from build123d import *

# Parameters (mm, degrees)
PAD_DEPTH        = 3
HOLE_D           = 3.5
HOLE_CSINK_D     = 7
HOLE_CSINK_ANGLE = 90
CHAMFER_SIZE     = 1
SKETCH002_W      = 31
SKETCH002_H      = 47
POCKET_DEPTH     = 2.2
SKETCH003_W      = 28
SKETCH003_H      = 47
POCKET001_DEPTH  = 3.001
POCKET002_DEPTH  = 3.001
CHAMFER001_SIZE  = 0.5
PAD001_DEPTH     = 15


with BuildPart() as part:
    # Sketch → Pad (new body)
    with BuildSketch(Plane.XY):
        with BuildLine():
            Line((6, 0), (46.1, 0))
            ThreePointArc((46.1, 0), (50.342641, 1.757359), (52.1, 6))
            Line((52.1, 6), (52.1, 62))
            ThreePointArc((52.1, 62), (50.342641, 66.242641), (46.1, 68))
            Line((46.1, 68), (6, 68))
            ThreePointArc((6, 68), (1.757359, 66.242641), (0, 62))
            Line((0, 62), (0, 6))
            ThreePointArc((0, 6), (1.757359, 1.757359), (6, 0))
        make_face()
    extrude(amount=PAD_DEPTH)

    # Hole (through all)
    with Locations(Plane(origin=(0, 0, 0), x_dir=(1, 0, 0), z_dir=(0, 0, -1))):
        with Locations((6, -52.65), (46.1, -52.65), (46.1, -15.35), (6, -15.35)):
            CounterSinkHole(HOLE_D / 2, HOLE_CSINK_D / 2, counter_sink_angle=HOLE_CSINK_ANGLE)

    # Chamfer
    chamfer_edges = [part.edges().sort_by_distance(p)[0] for p in [
        (52.1, 34, 0),
    ]]
    chamfer(chamfer_edges, length=CHAMFER_SIZE)

    # Sketch002 (on DatumPlane) → Pocket (cut)
    with BuildSketch(Plane.XY.offset(3)):
        with Locations((26.05, 27)):
            Rectangle(SKETCH002_W, SKETCH002_H)
    extrude(amount=-POCKET_DEPTH, mode=Mode.SUBTRACT)

    # Sketch003 (on DatumPlane) → Pocket001 (cut, through all)
    with BuildSketch(Plane.XY.offset(3)):
        with Locations((26.05, 27)):
            Rectangle(SKETCH003_W, SKETCH003_H)
    extrude(amount=-POCKET001_DEPTH, mode=Mode.SUBTRACT)

    # Sketch004 (on DatumPlane) → Pocket002 (cut, through all)
    with BuildSketch(Plane.XY.offset(3)):
        with BuildLine():
            Line((11.05, 54.5), (11.05, 65.5))
            ThreePointArc((11.55, 66), (11.196447, 65.853553), (11.05, 65.5))
            Line((11.55, 66), (40.55, 66))
            ThreePointArc((41.05, 65.5), (40.903553, 65.853553), (40.55, 66))
            Line((41.05, 65.5), (41.05, 54.5))
            ThreePointArc((40.55, 54), (40.903553, 54.146447), (41.05, 54.5))
            Line((40.55, 54), (11.55, 54))
            ThreePointArc((11.05, 54.5), (11.196447, 54.146447), (11.55, 54))
        make_face()
    extrude(amount=-POCKET002_DEPTH, mode=Mode.SUBTRACT)

    # Chamfer001
    chamfer001_edges = [part.edges().sort_by_distance(p)[0] for p in [
        (26.05, 54, 0),
        (26.05, 54, 3),
    ]]
    chamfer(chamfer001_edges, length=CHAMFER001_SIZE)

    # Sketch005 (on DatumPlane) → Pad001 (join)
    with BuildSketch(Plane.XY.offset(3)):
        with BuildLine():
            Line((10.05, 52.5), (10.05, 51.5))
            ThreePointArc((10.05, 51.5), (10.342893, 50.792893), (11.05, 50.5))
            Line((11.05, 50.5), (41.05, 50.5))
            ThreePointArc((41.05, 50.5), (41.757107, 50.792893), (42.05, 51.5))
            Line((42.05, 51.5), (42.05, 52.5))
            ThreePointArc((42.05, 52.5), (41.757107, 53.207107), (41.05, 53.5))
            Line((41.05, 53.5), (11.05, 53.5))
            ThreePointArc((11.05, 53.5), (10.342893, 53.207107), (10.05, 52.5))
        make_face()
    extrude(amount=PAD001_DEPTH)


solid = part.part
Verification items for the finished model (mm, model axes). A direction names the side the tool comes from. Give positions to 0.01 mm unless a question says otherwise; leave off trailing zeros. Write each loop counter-clockwise with the first axis right and the second up, starting at its lowest first coordinate (ties: lowest second). Pieces come first, ordered by that corner, then holes. Notation, with made-up numbers: M 66.5,35.5 L 109.5,35.5 A18 cw 109.5,57.5 Z; hole C 44.25,45.25 d6. An arc over 180 degrees is marked long. Use CSV: the item, a comma, the result in double quotes.
1) Cross-section at C-C (z = 9). Enter the section's corners in (x, y).
Final values:
outline,"M 10.05,51.5 A1 ccw 11.05,50.5 L 41.05,50.5 A1 ccw 42.05,51.5 L 42.05,52.5 A1 ccw 41.05,53.5 L 11.05,53.5 A1 ccw 10.05,52.5 Z"
2) Cross-section at A-A (x = 24). Enter the section's corners in (y, z), plus the area to 3 significant figures.
Final values:
outline,"M 0,1 L 1,0 L 3.5,0 L 3.5,3 L 0,3 Z; M 50.5,0 L 53.5,0 L 54,0.5 L 54,2.5 L 53.5,3 L 53.5,18 L 50.5,18 Z; M 66,0.5 L 66.5,0 L 67,0 L 68,1 L 68,3 L 66.5,3 L 66,2.5 Z"
area,"70.5 mm²"
3) Go/stop test with flat-tipped pins: pin 1 Ø1 at (x, y) = (45, 54) entering from +Z; pin 2 Ø8 at (y, z) = (47.5, 11.5) entering from +X; pin 3 Ø10 at (x, z) = (41.5, 14) entering from +Y; pin 4 Ø10 at (x, z) = (42.5, 7) entering from +Y. Record where each tip stops, or that it passes through.
Final values:
pin 1,"z = 3"
pin 2,"x = 42.05"
pin 3,"y = 53.5"
pin 4,"y = 68"
4) Release check for a two-part mould opening along X. For faces 4 (the face through (26, 68, 2)), 5 (the face through (49.868, 65.686, 0.271)), 6 (the face through (6.38, 54.36, 2.38)) record: released by +X, released by -X, zero draft, split by the parting line, or undercut.
Final values:
face 4,"zero draft"
face 5,"released by +X"
face 6,"undercut"
5) Material ranges on line 1 along X through (y, z) = (52.65, 2.15); line 2 along Y through (x, z) = (46.1, 2.2); line 3 along X through (y, z) = (15.35, 2.3), recorded low to high.
Final values:
line 1,"0 to 4.25, 7.75 to 44.35, 47.85 to 52.1"
line 2,"0 to 13.6, 17.1 to 50.9, 54.4 to 68"
line 3,"0 to 4.25, 7.75 to 10.55, 41.55 to 44.35, 47.85 to 52.1"
6) Access from +Z, -Z, +X, -X, +Y, -Y to the whole of each face (thin tool, end or side, straight path). Record for faces 1 (the face through (1.804, 66.289, 1.986)), 2 (the face through (26, 66, 2)), 3 (the face through (10.55, 27, 2)).
Final values:
face 1,"+Z, -Z, -X, +Y"
face 2,"+Z, -Z"
face 3,"+Z"
7) Cross-section at B-B (y = 15.35). Enter the section's corners in (x, z), plus the area to 3 significant figures.
Final values:
outline,"M 0,1 L 1,0 L 2.5,0 L 4.25,1.75 L 4.25,3 L 0,3 Z; M 7.75,1.75 L 9.5,0 L 12.05,0 L 12.05,0.8 L 10.55,0.8 L 10.55,3 L 7.75,3 Z; M 40.05,0 L 42.6,0 L 44.35,1.75 L 44.35,3 L 41.55,3 L 41.55,0.8 L 40.05,0.8 Z; M 47.85,1.75 L 49.6,0 L 51.1,0 L 52.1,1 L 52.1,3 L 47.85,3 Z"
area,"37.6 mm²"
